Geometry: final body of the model. Coordinates: model frame, mm. Face numbers are marked on the shaded views. A direction names the side the tool comes from. Round coordinates to 2 decimals unless told otherwise and drop trailing zeros. Write each loop counter-clockwise with the first axis right and the second up, starting at its lowest first coordinate (ties: lowest second). Pieces come first, ordered by that corner, then holes. Notation, with made-up numbers: (12, -36.75) - (49, -36.75) arc R23 cw to (49, -14.75) - close; hole circle Ø1 at (3.25, 22). An arc over 180 degrees is marked (long way). Write each question's results on one line, items separated by ' | '.
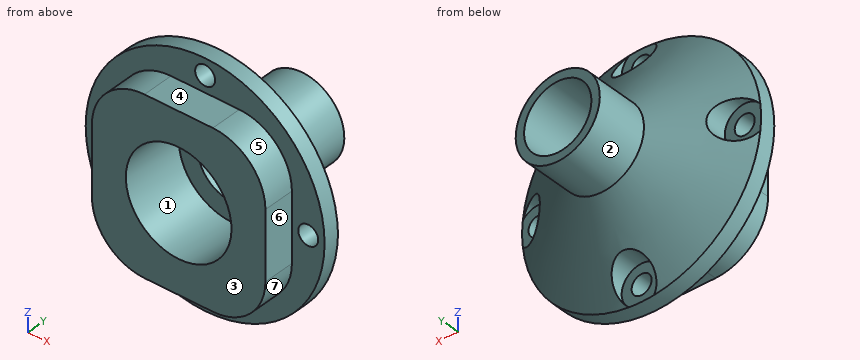
from build123d import *

# Parameters (mm, degrees)
CUT_EXTRUDE1_START = 3
SKETCH4_R          = 11.357
SKETCH4_R_2        = 0.95
CUT_EXTRUDE1_DEPTH = 3
CUT_EXTRUDE2_START = 18
SKETCH4_11_R       = 0.95
CUT_EXTRUDE2_DEPTH = 18
SKETCH5_R          = 1.9
CUT_EXTRUDE3_DEPTH = 6.875


with BuildPart() as part:
    # Sketch1 → Revolve1 (revolve)
    with BuildSketch(Plane.XY, mode=Mode.PRIVATE) as revolve1_sk:
        Polygon((-5.025, 0), (-11.357, 0), (-11.357, 4.5), (-4, 9), (-4, 14), (-3.2, 14), (-3.2, 6), (-5.025, 6), align=None)
    revolve(revolve1_sk.sketch.rotate(Axis((0, 0, 0), (0, 1, 0)), 270), axis=Axis((0, 0, 0), (0, 1, 0)))

    # Sketch4 → Cut-Extrude1 (cut)
    with BuildSketch(Plane(origin=(0, 0, 0), x_dir=(1, 0, 0), z_dir=(0, 1, 0)).offset(CUT_EXTRUDE1_START)):
        with Locations(Location((0, 0, 0), (0, 0, 90))):
            Circle(SKETCH4_R)
        with Locations(Location((-9.8035, 0, 0), (0, 0, 270))):
            Circle(SKETCH4_R_2, mode=Mode.SUBTRACT)
        with Locations(Location((0, -9.8035, 0), (0, 0, 270))):
            Circle(SKETCH4_R_2, mode=Mode.SUBTRACT)
        with BuildLine():
            ThreePointArc((-8.25, 3.25), (-6.785533906, 6.785533906), (-3.25, 8.25))
            Line((-3.25, 8.25), (0.661635478, 8.25))
            Line((0.661635478, 8.25), (3.25, 8.25))
            ThreePointArc((3.25, 8.25), (6.785533906, 6.785533906), (8.25, 3.25))
            Line((8.25, 3.25), (8.25, 0.661635478))
            Line((8.25, 0.661635478), (8.25, -3.25))
            ThreePointArc((8.25, -3.25), (6.785533906, -6.785533906), (3.25, -8.25))
            Line((3.25, -8.25), (-3.25, -8.25))
            ThreePointArc((-3.25, -8.25), (-6.785533906, -6.785533906), (-8.25, -3.25))
            Line((-8.25, -3.25), (-8.25, 0.661635478))
            Line((-8.25, 0.661635478), (-8.25, 3.25))
        make_face(mode=Mode.SUBTRACT)
        with Locations(Location((9.8035, 0, 0), (0, 0, 270))):
            Circle(SKETCH4_R_2, mode=Mode.SUBTRACT)
        with Locations(Location((0, 9.8035, 0), (0, 0, 270))):
            Circle(SKETCH4_R_2, mode=Mode.SUBTRACT)
    extrude(amount=-CUT_EXTRUDE1_DEPTH, mode=Mode.SUBTRACT)

    # Sketch4<11> → Cut-Extrude2 (cut)
    with BuildSketch(Plane(origin=(0, 0, 0), x_dir=(1, 0, 0), z_dir=(0, 1, 0)).offset(CUT_EXTRUDE2_START)):
        with Locations(Location((0, 9.8035, 0), (0, 0, 90.000000426))):
            Circle(SKETCH4_11_R)
        with Locations(Location((9.8035, 0, 0), (0, 0, 108.098639854))):
            Circle(SKETCH4_11_R)
        with Locations(Location((0, -9.8035, 0), (0, 0, 161.901360146))):
            Circle(SKETCH4_11_R)
        with Locations(Location((-9.8035, 0, 0), (0, 0, 149.382227185))):
            Circle(SKETCH4_11_R)
    extrude(amount=-CUT_EXTRUDE2_DEPTH, mode=Mode.SUBTRACT)

    # Sketch5 → Cut-Extrude3 (cut)
    with BuildSketch(Plane(origin=(0, 11.375, 0), x_dir=(1, 0, 0), z_dir=(0, 1, 0))):
        with Locations((0, 9.8125)):
            Circle(SKETCH5_R)
        with Locations((9.8125, 0)):
            Circle(SKETCH5_R)
        with Locations((0, -9.8125)):
            Circle(SKETCH5_R)
        with Locations((-9.8125, 0)):
            Circle(SKETCH5_R)
    extrude(amount=-CUT_EXTRUDE3_DEPTH, mode=Mode.SUBTRACT)


solid = part.part
Q1. Access query for the marked faces 5, 6 and 7. Directions: +Z, -Z, +X, -X, +Y, -Y. A direction counts if a zero-diameter tool reaches every point of the face in a straight line with its end or side. Return the directions, or none.
Answer block:
face 5: +Z, +X, -Y | face 6: +Z, -Z, +X, -Y | face 7: -Z, +X, -Y
Q2. Section query D-D, the plane y = 7. Return loops of the section in (x, z).
Answer block:
outline: circle Ø14.54 at (0, 0); hole circle Ø6.4 at (0, 0)
Q3. Section query A-A, the plane z = 0. Give the number of separate pieces and of enclosed holes in the cut face, plus the area to 3 significant figures.
Answer block:
separate pieces: 4 | enclosed holes: 0 | area: 68.2 mm2
Q4. Mould query, pull axis Z, two halves, no side actions, for the marked faces 1, 2, 3 and 4. Classes: pulls with the +Z half, pulls with the -Z half, needs draft (parallel to the pull), parting line crosses it, or undercut.
Answer block:
face 1: undercut | face 2: parting line crosses it | face 3: needs draft | face 4: pulls with the +Z half
Q5. Section query C-C, the plane y = 2.5. Return loops of the section in (x, z) (3 decimals).
Answer block:
outline: (-8.25, -3.25) arc R5 ccw to (-3.25, -8.25) - (3.25, -8.25) arc R5 ccw to (8.25, -3.25) - (8.25, 3.25) arc R5 ccw to (3.25, 8.25) - (-3.25, 8.25) arc R5 ccw to (-8.25, 3.25) - close; hole circle Ø10.05 at (0, 0)
Q6. Ray query, line 1 along X through (y, z) = (10.5, 0); line 2 along X through (y, z) = (2.2, 0) (3 decimals); line 3 along Z through (x, y) = (-1.75, 3.75). Return the intervals inside material, ascending.
Answer block:
line 1: -4 to -3.2, 3.2 to 4 | line 2: -8.25 to -5.025, 5.025 to 8.25 | line 3: -11.22 to -4.71, 4.71 to 11.22
Q7. Pin query (flat end, axial travel): pin 1 (3 mm diameter, centred on x = 0, z = 9.8, fed in from -Y); pin 2 (3 mm diameter, centred on x = -5.5, y = 5.5, fed in from +Z); pin 3 (1 mm diameter, centred on x = 1, z = 10, fed in from +Y); pin 4 (13 mm diameter, centred on x = 0, z = 0, fed in from +Y). Return the tip coordinate at first contact, or that it passes through.
Answer block:
pin 1: y = 3 | pin 2: z = 10.48 | pin 3: y = 4.5 | pin 4: y = 14
